from build123d import *

# Parameters (mm, degrees)
SKETCH1_W           = 119
SKETCH1_H           = 104
BOSS_EXTRUDE1_DEPTH = 10
SKETCH2_W           = 35
SKETCH2_H           = 25
CUT_EXTRUDE1_DEPTH  = 80.650800373
SKETCH3_W           = 34
SKETCH3_H           = 70
CUT_EXTRUDE2_DEPTH  = 8
SKETCH4_W           = 77
SKETCH4_H           = 81
CUT_EXTRUDE3_DEPTH  = 8
CUT_EXTRUDE4_DEPTH  = 10
SKETCH7_W           = 10
SKETCH7_H           = 10
CUT_EXTRUDE6_DEPTH  = 2


with BuildPart() as part:
    # Sketch1 → Boss-Extrude1 (new body)
    with BuildSketch(Plane(origin=(0, 0, 0), x_dir=(1, 0, 0), z_dir=(0, 1, 0))):
        Rectangle(SKETCH1_W, SKETCH1_H)
    extrude(amount=BOSS_EXTRUDE1_DEPTH)

    # Sketch2 → Cut-Extrude1 (cut, through all)
    with BuildSketch(Plane(origin=(0, 10, 0), x_dir=(1, 0, 0), z_dir=(0, 1, 0))):
        with Locations((42, -39.5)):
            Rectangle(SKETCH2_W, SKETCH2_H)
    extrude(amount=-CUT_EXTRUDE1_DEPTH, mode=Mode.SUBTRACT)

    # Sketch3 → Cut-Extrude2 (cut)
    with BuildSketch(Plane(origin=(0, 10, 0), x_dir=(1, 0, 0), z_dir=(0, 1, 0))):
        with Locations((40.5, 10)):
            Rectangle(SKETCH3_W, SKETCH3_H)
    extrude(amount=-CUT_EXTRUDE2_DEPTH, mode=Mode.SUBTRACT)

    # Sketch4 → Cut-Extrude3 (cut)
    with BuildSketch(Plane(origin=(0, 10, 0), x_dir=(1, 0, 0), z_dir=(0, 1, 0))):
        with Locations((-17, -9.5)):
            Rectangle(SKETCH4_W, SKETCH4_H)
    extrude(amount=-CUT_EXTRUDE3_DEPTH, mode=Mode.SUBTRACT)

    # Sketch5 → Cut-Extrude4 (cut)
    with BuildSketch(Plane(origin=(0, 10, 0), x_dir=(1, 0, 0), z_dir=(0, 1, 0))):
        Polygon((-59.5, 52), (59.5, 52), (59.5, 47), (21.5, 47), (21.5, 33), (-57.5, 33), (-57.5, -52), (-59.5, -52), align=None)
    extrude(amount=-CUT_EXTRUDE4_DEPTH, mode=Mode.SUBTRACT)

    # Sketch7 → Cut-Extrude6 (cut)
    with BuildSketch(Plane.ZY.offset(57.5)):
        with Locations((-13, 5)):
            Rectangle(SKETCH7_W, SKETCH7_H)
    extrude(amount=-CUT_EXTRUDE6_DEPTH, mode=Mode.SUBTRACT)


solid = part.part
Work out the finished part from the listing and answer in its coordinate system (mm). A direction names the side the tool comes from. Coordinates: 2 decimals unless noted, no trailing zeros. Loops run counter-clockwise (first coordinate to the right, second up) from the corner with the lowest first, then second, coordinate; pieces in that order, holes last. Notation, with made-up numbers: (11, -7.5) -> (62, -7.5) arc R23 cw to (62, 6.5) -> close; hole circle Ø5 at (83, 19). An arc over 180 degrees is marked (long way). Answer as CSV lines item,"result".
1) For faces 4 (the face through (57.5, 6, -10)), 5 (the face through (42, 5, 27)), 6 (the face through (22, 10, -1)), 7 (the face through (21.5, 5, -40)), determine the directions among +Z, -Z, +X, -X, +Y, -Y from which every point of the face is accessible in a straight line to the end or side of a thin tool.
A:
face 4,"+Y"
face 5,"+Z, +X, +Y, -Y"
face 6,"+Z, -Z, +X, -X, +Y"
face 7,"-Z, -X, +Y, -Y"
2) Straight lines are drawn through the part: probe 1 along X at (y, z) = (4, 12); probe 2 along Z at (x, y) = (-21, 8); probe 3 along X at (y, z) = (7.75, 42). For each, find the intervals that lie inside material, in ascending order.
A:
probe 1,"x = -57.5 to -55.5, 21.5 to 23.5, 57.5 to 59.5"
probe 2,"z = -33 to -31, 50 to 52"
probe 3,"x = -57.5 to -55.5, 21.5 to 24.5"
3) Flat-ended cylindrical pins translate along their axes: pin 1 (4 mm diameter, centred on x = 38.5, y = 4.5, fed in from +Z); pin 2 (0.6 mm diameter, centred on x = -56.5, y = 5, fed in from -Z); pin 3 (3 mm diameter, centred on y = 6.5, z = 42, fed in from +X). Find the tip coordinate at first contact, or state that the pin passes through.
A:
pin 1,"stops at z = 27"
pin 2,"stops at z = -33"
pin 3,"stops at x = 24.5"
4) The part is cut by section D-D (x = 31). Give the vertices of the cut face in (y, z).
A:
outline,"(0, -47) -> (10, -47) -> (10, -45) -> (2, -45) -> (2, 25) -> (10, 25) -> (10, 27) -> (0, 27) -> close"
5) The part is cut by section A-A (x = -39). Give the vertices of the cut face in (y, z).
A:
outline,"(0, -33) -> (10, -33) -> (10, -31) -> (2, -31) -> (2, 50) -> (10, 50) -> (10, 52) -> (0, 52) -> close"
6) The part is cut by section C-C (y = 5). Give the vertices of the cut face in (x, z), and give its area (3 significant figures).
A:
outline,"(-57.5, -33) -> (21.5, -33) -> (21.5, -47) -> (59.5, -47) -> (59.5, 27) -> (24.5, 27) -> (24.5, 52) -> (-57.5, 52) -> (-57.5, -8) -> (-55.5, -8) -> (-55.5, 50) -> (21.5, 50) -> (21.5, -31) -> (-55.5, -31) -> (-55.5, -18) -> (-57.5, -18) -> close; hole (23.5, -45) -> (57.5, -45) -> (57.5, 25) -> (23.5, 25) -> close"
area,"965 mm²"
7) For a pull along X with two mould halves and no side action, classify faces 1 (the face through (24.5, 5, 40)), 2 (the face through (-18, 2, 9)), 3 (the face through (41, 5, -47)) as released by +X, released by -X, zero draft, split by the parting line, or undercut.
A:
face 1,"released by +X"
face 2,"undercut"
face 3,"zero draft"
8) The part is cut by section B-B (z = 2). Give the vertices of the cut face in (x, y).
A:
outline,"(-57.5, 0) -> (59.5, 0) -> (59.5, 10) -> (57.5, 10) -> (57.5, 2) -> (23.5, 2) -> (23.5, 10) -> (21.5, 10) -> (21.5, 2) -> (-55.5, 2) -> (-55.5, 10) -> (-57.5, 10) -> close"
